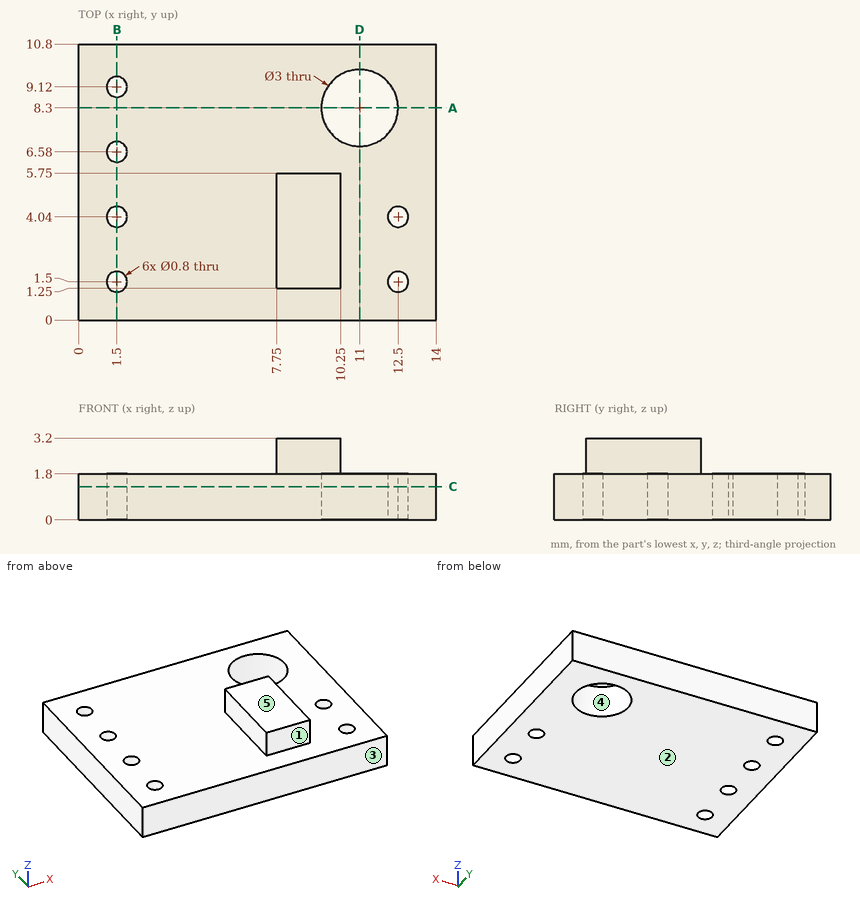
Job drawing, mm, ordinate dimensions from the low corner. One solid piece. A direction names the side the tool comes from. Coordinates: 2 decimals unless noted, no trailing zeros. Write each loop counter-clockwise with the first axis right and the second up, starting at its lowest first coordinate (ties: lowest second). Pieces come first, ordered by that corner, then holes. Notation, with made-up numbers: (-0.75, 25) -> (20.25, 25) arc R22 cw to (20.25, 50) -> close; hole circle Ø11 at (65.5, 86). An arc over 180 degrees is marked (long way). Use CSV: the item, a comma, the result in double quotes. Start each with the question number.
Item 1: Band-saw the part on D-D, the plane x = 11. Write the cut outline in (y, z), plus the area to 3 significant figures.
Item 2: Two-plate mould, pull along Y, no slides. Class the marked faces 3, 4 and 5: +Y half, -Y half, draft (parallel to the pull), parting line (faces both ways), or undercut.
Item 3: Band-saw the part on C-C, the plane z = 1.3. Write the cut outline in (x, y).
Item 4: Drop flat-ended pins along their axis: P1, Ø0.7, axis at y = 3.5, z = 2.5, coming from the +X side; P2, Ø1.1, axis at x = 8.5, z = 2.5, coming from the +Y side; P3, Ø2.5, axis at x = 11, y = 8.3, coming from the +Z side; P4, Ø2, axis at x = 9.5, y = 9.5, coming from the +Z side. Give the stop position or say it passes through.
Item 5: Wall check: probe 1 along Y at (x, z) = (1.5, 0.45); probe 2 along X at (y, z) = (4, 1.7); probe 3 along X at (y, z) = (1.75, 1.15). Give the ranges that are in metal, low to high.
Item 6: Band-saw the part on A-A, the plane y = 8.3. Write the cut outline in (x, z).
Item 7: Band-saw the part on B-B, the plane x = 1.5. Write the cut outline in (y, z).
Item 8: Tool access for the marked faces 1 and 2: list every direction of +Z, -Z, +X, -X, +Y, -Y with a clear straight run to the whole face (end or side of a thin tool).
Response values:
1,outline,"(0, 0) -> (6.8, 0) -> (6.8, 1.8) -> (0, 1.8) -> close; (9.8, 0) -> (10.8, 0) -> (10.8, 1.8) -> (9.8, 1.8) -> close"
1,area,"14.0 mm2"
2,face 3,"-Y half"
2,face 4,"undercut"
2,face 5,"draft"
3,outline,"(0, 0) -> (14, 0) -> (14, 10.8) -> (0, 10.8) -> close; hole circle Ø0.8 at (1.5, 1.5); hole circle Ø0.8 at (1.5, 4.04); hole circle Ø0.8 at (1.5, 6.58); hole circle Ø0.8 at (1.5, 9.12); hole circle Ø3 at (11, 8.3); hole circle Ø0.8 at (12.5, 1.5); hole circle Ø0.8 at (12.5, 4.04)"
4,P1,"stops at x = 10.25"
4,P2,"stops at y = 5.75"
4,P3,"passes through"
4,P4,"stops at z = 1.8"
5,probe 1,"y = 0 to 1.1, 1.9 to 3.64, 4.44 to 6.18, 6.98 to 8.72, 9.52 to 10.8"
5,probe 2,"x = 0 to 1.1, 1.9 to 12.1, 12.9 to 14"
5,probe 3,"x = 0 to 1.19, 1.81 to 12.19, 12.81 to 14"
6,outline,"(0, 0) -> (9.5, 0) -> (9.5, 1.8) -> (0, 1.8) -> close; (12.5, 0) -> (14, 0) -> (14, 1.8) -> (12.5, 1.8) -> close"
7,outline,"(0, 0) -> (1.1, 0) -> (1.1, 1.8) -> (0, 1.8) -> close; (1.9, 0) -> (3.64, 0) -> (3.64, 1.8) -> (1.9, 1.8) -> close; (4.44, 0) -> (6.18, 0) -> (6.18, 1.8) -> (4.44, 1.8) -> close; (6.98, 0) -> (8.72, 0) -> (8.72, 1.8) -> (6.98, 1.8) -> close; (9.52, 0) -> (10.8, 0) -> (10.8, 1.8) -> (9.52, 1.8) -> close"
8,face 1,"+Z, +X, -X, -Y"
8,face 2,"-Z, +X, -X, +Y, -Y"
